Design review of the part shown in the three views and the two pictorial views. Dimensions are in mm from the part's minimum x, y and z. A direction names the side the tool comes from. Give positions to 0.01 mm unless a question says otherwise; leave off trailing zeros. Loops run counter-clockwise (first coordinate to the right, second up) from the corner with the lowest first, then second, coordinate; pieces in that order, holes last. Notation, with made-up numbers: (-9, -32) - (2, -32) arc R36 cw to (2, 2) - close; hole circle Ø3 at (-2, -15). An arc over 180 degrees is marked (long way). Answer as a JSON object with one key per item and string values.
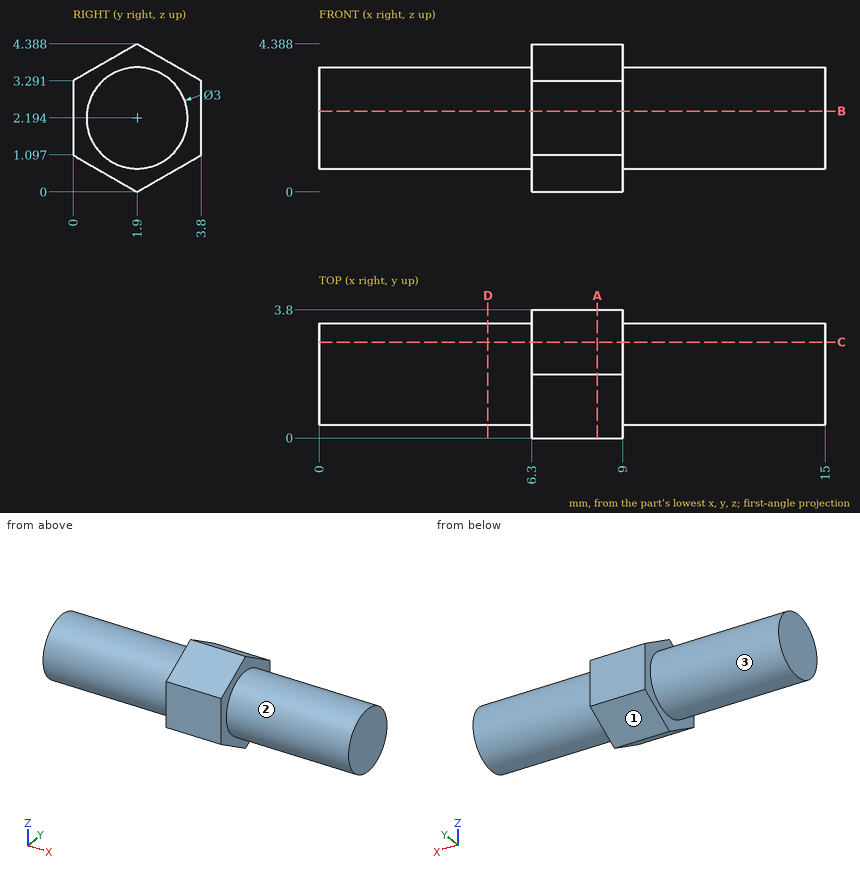
Q1. Consider section D-D, the plane x = 5. State the section outline as (y, z) points, plus the area to 3 significant figures.
Results:
{"outline": "circle Ø3 at (1.9, 2.19)", "area": "7.07 mm^2"}
Q2. For the marked faces 1, 2 and 3, list the 3-axis set-ups (+Z, -Z, +X, -X, +Y, -Y) from which the entire face can be reached by the end or side of a thin tool; tool diameter is ignored.
Results:
{"face 1": "-Z, +X, -X, +Y", "face 2": "+X", "face 3": "-X"}
Q3. To check wall thickness, follow probe 1 along Z at (x, y) = (3.75, 2); probe 2 along X at (y, z) = (3.25, 3.05); probe 3 along Y at (x, z) = (2.75, 1.1). State the ranges of each line that lie inside material, in increasing order. Write a range as [from, to].
Results:
{"probe 1": "z = [0.7, 3.69]", "probe 2": "x = [6.3, 9]", "probe 3": "y = [0.87, 2.93]"}
Q4. Clearance check with a flat-ended pin moving along its axis: pin 1 Ø2 at (x, z) = (12, 2.5) entering from +Y. State where the tip first meets the part, or that it passes through.
Results:
{"pin 1": "stops at y = 3.4"}
Q5. Consider section B-B, the plane z = 2.4. State the section outline as (x, y) points, plus the area to 3 significant figures.
Results:
{"outline": "(0, 0.41) - (6.3, 0.41) - (6.3, 0) - (9, 0) - (9, 0.41) - (15, 0.41) - (15, 3.39) - (9, 3.39) - (9, 3.8) - (6.3, 3.8) - (6.3, 3.39) - (0, 3.39) - close", "area": "46.8 mm^2"}
Q6. Consider section C-C, the plane y = 2.85. State the section outline as (x, z) points (1 decimal).
Results:
{"outline": "(0, 1) - (6.3, 1) - (6.3, 0.5) - (9, 0.5) - (9, 1) - (15, 1) - (15, 3.4) - (9, 3.4) - (9, 3.8) - (6.3, 3.8) - (6.3, 3.4) - (0, 3.4) - close"}
Q7. Consider section A-A, the plane x = 8.25. State the section outline as (y, z) points.
Results:
{"outline": "(0, 1.1) - (1.9, 0) - (3.8, 1.1) - (3.8, 3.29) - (1.9, 4.39) - (0, 3.29) - close"}
